Source: CAD feature listing. Evaluate the final solid. Frame: model axes, mm. A direction names the side the tool comes from. Give positions to 0.01 mm unless a question says otherwise; leave off trailing zeros. Loops run counter-clockwise (first coordinate to the right, second up) from the corner with the lowest first, then second, coordinate; pieces in that order, holes last. Notation, with made-up numbers: (65.5, -22) -> (94.5, -22) arc R18 ccw to (94.5, 8) -> close; hole circle Ø10 at (6.5, 55.5). An arc over 180 degrees is marked (long way). Return JSON: item names as keys, results as strings. Group by question number.
(1) Draft query along Y for faces 1 (the face through (15.45, 3.71, 84.38)), 2 (the face through (13.5, 0, -1)), 3 (the face through (27.5, -3.92, 1.42)). Return one class per face: released by +Y, released by -Y, zero draft, split by the parting line, or undercut.
(2) Pin query (flat end, axial travel): pin 1 (3 mm diameter, centred on x = 18, y = 50, fed in from -Z); pin 2 (1.6 mm diameter, centred on x = 22.5, y = 0.5, fed in from -Z); pin 3 (3.5 mm diameter, centred on y = -0.5, z = -0.5, fed in from +X). Return the tip coordinate at first contact, or that it passes through.
(3) Cut plane A-A on z = 0. Return loops of the section in (x, y), then the cut area to 3 significant figures.
(4) Cut plane C-C on x = -3. Return loops of the section in (y, z), then the cut area to 3 significant figures.
(5) Access query for faces 4 (the face through (-15.45, 3.71, 84.38)), 5 (the face through (21, 0, 3)). Directions: +Z, -Z, +X, -X, +Y, -Y. A direction counts if a zero-diameter tool reaches every point of the face in a straight line with its end or side. Return the directions, or none.
(6) Ray query, line 1 (X direction, y = -12, z = -12); line 2 (Y direction, x = 17, z = 0); line 3 (Y direction, x = 19.75, z = 0). Return the intervals inside material, ascending. Write a range as from..to.
(7) Cut plane B-B on x = -16.5. Return loops of the section in (y, z).
```python
from build123d import *

# Parameters (mm, degrees)
SKETCH1_R                     = 85
BOSS_EXTRUDE1_DEPTH           = 25
BOSS_EXTRUDE1_TAPER           = 2
BOSS_EXTRUDE1_OTHER_WAY_DEPTH = 25
BOSS_EXTRUDE1_OTHER_WAY_TAPER = 2
SKETCH2_R                     = 6
BOSS_EXTRUDE2_DEPTH           = 2.5
CUT_EXTRUDE1_DEPTH            = 14


with BuildPart() as part:
    # Sketch1 → Boss-Extrude1 (new body)
    with BuildSketch(Plane(origin=(0, 0, 0), x_dir=(0, 0, -1), z_dir=(1, 0, 0))):
        Circle(SKETCH1_R)
    extrude(amount=BOSS_EXTRUDE1_DEPTH, taper=BOSS_EXTRUDE1_TAPER)

    # Sketch1 → Boss-Extrude1 other way (add)
    with BuildSketch(Plane(origin=(0, 0, 0), x_dir=(0, 0, -1), z_dir=(1, 0, 0))):
        Circle(SKETCH1_R)
    extrude(amount=-BOSS_EXTRUDE1_OTHER_WAY_DEPTH, taper=BOSS_EXTRUDE1_OTHER_WAY_TAPER)

    # Sketch2 → Boss-Extrude2 (add)
    with BuildSketch(Plane(origin=(25, 0, 0), x_dir=(0, 0, -1), z_dir=(1, 0, 0))):
        Circle(SKETCH2_R)
    extrude(amount=BOSS_EXTRUDE2_DEPTH)

    # Sketch3 → Cut-Extrude1 (cut)
    with BuildSketch(Plane(origin=(27.5, 0, 0), x_dir=(0, 0, -1), z_dir=(1, 0, 0))):
        with BuildLine():
            Line((-3, -2.645751311), (-3, 2.645751311))
            ThreePointArc((-3, 2.645751311), (4, 0), (-3, -2.645751311))
        make_face()
    extrude(amount=-CUT_EXTRUDE1_DEPTH, mode=Mode.SUBTRACT)


solid = part.part
```
Answers:
{
 "1": {"face 1": "split by the parting line", "face 2": "undercut", "face 3": "zero draft"},
 "2": {"pin 1": "z = -69.04", "pin 2": "z = -84.24", "pin 3": "x = 13.5"},
 "3": {"outline": "(-25, -84.13) -> (0, -85) -> (25, -84.13) -> (25, -6) -> (27.5, -6) -> (27.5, -4) -> (13.5, -4) -> (13.5, 4) -> (27.5, 4) -> (27.5, 6) -> (25, 6) -> (25, 84.13) -> (0, 85) -> (-25, 84.13) -> close", "area": "8,370 mm²"},
 "4": {"outline": "circle Ø169.79 at (0, 0)", "area": "22,600 mm²"},
 "5": {"face 4": "-X", "face 5": "+X"},
 "6": {"line 1": "-25..25", "line 2": "-84.41..-4, 4..84.41", "line 3": "-84.31..-4, 4..84.31"},
 "7": {"outline": "circle Ø168.85 at (0, 0)"}
}
